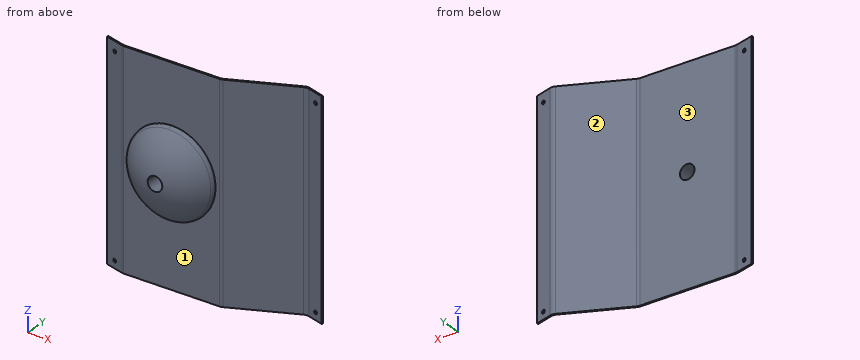
```python
from build123d import *

# Parameters (mm, degrees)
BOSS_EXTRUDE1_DEPTH = 290
SKETCH2_R           = 60
BOSS_EXTRUDE2_DEPTH = 5
DOME1_FACE_RADIUS   = 60
DOME1_HEIGHT        = 30
FILLET1_R           = 10
SKETCH3_R           = 10
CUT_EXTRUDE1_DEPTH  = 335.423734017
FILLET2_R           = 10
FILLET3_R           = 10
SKETCH8_R           = 2.42
SKETCH8_R_2         = 2.420000001
CUT_EXTRUDE2_DEPTH  = 40


with BuildPart() as part:
    # Sketch1 → Boss-Extrude1 (new body)
    with BuildSketch(Plane.XY):
        Polygon((0, 0), (-135, 0), (-161.533498532, 7.226579802), (-161.007929092, 9.156288786), (-134.732514829, 2), (-0.434386742, 2), (88.562311317, 42.572930951), (114.981959712, 34.864758374), (114.421796177, 32.944806079), (88.715656235, 40.444806079), align=None)
    extrude(amount=BOSS_EXTRUDE1_DEPTH)

    # Sketch2 → Boss-Extrude2 (add)
    with BuildSketch(Plane(origin=(0, 2, 0), x_dir=(1, 0, 0), z_dir=(0, 1, 0))):
        with Locations(Location((-67.583450785, -149.769450313, 0), (0, 0, 270))):
            Circle(SKETCH2_R)
    extrude(amount=-BOSS_EXTRUDE2_DEPTH)

    # Dome1: a dome of height H over a round flat face of radius A is a cap of a sphere of radius (A * A + H * H) / (2 * H)
    dome1_r = (DOME1_FACE_RADIUS * DOME1_FACE_RADIUS + DOME1_HEIGHT * DOME1_HEIGHT) / (2 * DOME1_HEIGHT)
    dome1_base = Plane((-67.583450785, -3, 149.769450313), z_dir=(0, -1, 0))
    with Locations(dome1_base.offset(DOME1_HEIGHT - dome1_r)):
        dome1_ball = Sphere(dome1_r, mode=Mode.PRIVATE)
    add(split(dome1_ball, bisect_by=dome1_base, keep=Keep.TOP, mode=Mode.PRIVATE))

    # Fillet1
    # the kernel refuses this fillet: 10 mm, written as the material it takes off along each edge
    with BuildSketch(Plane(origin=(-67.583450785, -3, 149.769450313), x_dir=(4.089410291877963e-12, 0, -1.0), z_dir=(1.0, 0, 4.089410291877963e-12))) as fillet1_piece_1:
        with BuildLine():
            CenterArc((50.011565498, 3.480807854), FILLET1_R, 320.300820282, 36.943291115)
            Line((57.705652497, -2.906760168), (57.859534237, -3.034511529))
            ThreePointArc((57.859534237, -3.034511529), (59.02775796, -1.591456193), (60.16, -0.12))
            Line((60.16, -0.12), (60.2, 0))
            ThreePointArc((60.2, 0), (60.2, 1.5), (60.19976869, 2.990383843))
            Line((60.19976869, 2.990383843), (60, 3))
        make_face()
    revolve(axis=Axis((-67.583450785, -3, 149.769450313), (0, 1, 0)), revolution_arc=180, mode=Mode.SUBTRACT)
    with BuildSketch(Plane(origin=(-67.583450785, -3, 149.769450313), x_dir=(0, 0, 1), z_dir=(-1, 0, 0))) as fillet1_piece_2:
        with BuildLine():
            CenterArc((50.011565498, 3.480807853), FILLET1_R, 320.300820281, 36.94329112)
            Line((57.705652497, -2.906760169), (57.859534237, -3.03451153))
            ThreePointArc((57.859534237, -3.03451153), (59.02775796, -1.591456194), (60.16, -0.12))
            Line((60.16, -0.12), (60.2, 0))
            ThreePointArc((60.2, 0), (60.2, 1.5), (60.19976869, 2.990383843))
            Line((60.19976869, 2.990383843), (60, 3))
        make_face()
    revolve(axis=Axis((-67.583450785, -3, 149.769450313), (0, 1, 0)), revolution_arc=180, mode=Mode.SUBTRACT)

    # Sketch3 → Cut-Extrude1 (cut, through all)
    with BuildSketch(Plane(origin=(0, 2, 0), x_dir=(1, 0, 0), z_dir=(0, 1, 0))):
        with Locations(Location((-67.583450785, -149.769450313, 0), (0, 0, 270))):
            Circle(SKETCH3_R)
    extrude(amount=-CUT_EXTRUDE1_DEPTH, mode=Mode.SUBTRACT)

    # Fillet2
    fillet2_edges = [part.edges().sort_by_distance(p)[0] for p in [
        (88.562311317, 42.572930951, 145),
        (88.715656235, 40.444806079, 145),
    ]]
    fillet(fillet2_edges, radius=FILLET2_R)

    # Fillet3
    fillet3_edges = [part.edges().sort_by_distance(p)[0] for p in [
        (0, 0, 145),
        (-135, 0, 145),
        (-134.732514829, 2, 145),
        (-0.434386742, 2, 145),
    ]]
    fillet(fillet3_edges, radius=FILLET3_R)

    # Sketch8 → Cut-Extrude2 (cut)
    with BuildSketch(Plane(origin=(0, 0, 0), x_dir=(1, 0, 0), z_dir=(0, 1, 0))):
        with Locations((-148.387339129, -10.01871293)):
            Circle(SKETCH8_R)
        with Locations((103.912660871, -10.01871293)):
            Circle(SKETCH8_R)
        with Locations((103.912660871, -276.91871293)):
            Circle(SKETCH8_R)
        with Locations((-148.387339129, -276.91871293)):
            Circle(SKETCH8_R_2)
    extrude(amount=CUT_EXTRUDE2_DEPTH, mode=Mode.SUBTRACT)


solid = part.part
```
Model file for the job. Use its own axes, mm. Face numbers are marked on the shaded views. Coordinates: 2 decimals unless noted, no trailing zeros. Write each loop counter-clockwise with the first axis right and the second up, starting at its lowest first coordinate (ties: lowest second). Pieces come first, ordered by that corner, then holes. Notation, with made-up numbers: (65, 15.25) - (85, 15.25) arc R36 cw to (85, 50.25) - close; hole circle Ø1 at (25.5, 18.5). An arc over 180 degrees is marked (long way). One line per question, with ' | ' between items. Start each with the question number.
Q1. Drill centre lines: line 1 (Y direction, x = -91, z = 66); line 2 (X direction, y = 30, z = 138.5); line 3 (Y direction, x = 38.5, z = 221). Where is each one in solid material? Low to high. Write a range as [from, to].
Q2. Cut at D-D, the plane x = 64. List the corners of the cut face in (y, z).
Q3. Pin check, flat tips, straight feed: pin 1 (7.5 mm diameter, centred on x = 103.91, z = 276.92, fed in from -Y); pin 2 (4 mm diameter, centred on y = 20.5, z = 192, fed in from -X); pin 3 (2 mm diameter, centred on y = 22.5, z = 135.5, fed in from +X). Stop position of each tip, or through.
Q4. Cut at C-C, the plane y = 13.5. List the corners of the cut face in (x, z).
Q5. Cut at B-B, the plane y = -10.5. List the corners of the cut face in (x, z), then the cut area to 3 significant figures.
Q6. Cut at A-A, the plane z = 72.5. List the corners of the cut face in (x, y).
Q7. Pull direction X, two halves, no side cores. Call the marked faces 1, 2 and 3: pulls with the +X half, pulls with the -X half, needs draft (parallel to the pull), parting line crosses it, or undercut.
Answer below:
1) line 1: [0, 2] | line 2: [60.98, 65.8] | line 3: [17.55, 19.75]
2) outline: (29.18, 0) - (31.38, 0) - (31.38, 290) - (29.18, 290) - close
3) pin 1: y = 34.92 | pin 2: x = 35.76 | pin 3: x = 51.55
4) outline: (24.79, 0) - (29.61, 0) - (29.61, 290) - (24.79, 290) - close
5) outline: circle Ø107.12 at (-67.58, 149.77); hole circle Ø20 at (-67.58, 149.77) | area: 8,700 mm^2
6) outline: (-161.53, 7.23) - (-136.29, 0.35) arc R10 ccw to (-133.66, 0) - (-2.17, 0) arc R10 ccw to (1.98, 0.9) - (85.33, 38.9) arc R10 cw to (92.28, 39.4) - (114.42, 32.94) - (114.98, 34.86) - (92.13, 41.53) arc R10 ccw to (85.18, 41.03) - (1.54, 2.9) arc R10 cw to (-2.61, 2) - (-133.4, 2) arc R10 cw to (-136.02, 2.35) - (-161.01, 9.16) - close
7) face 1: needs draft | face 2: undercut | face 3: undercut
